Could you check a few things on this model? Use its own coordinates, in mm. Face numbers are marked on the shaded views. A direction names the side the tool comes from. Round coordinates to 2 decimals unless told otherwise and drop trailing zeros. Loops run counter-clockwise (first coordinate to the right, second up) from the corner with the lowest first, then second, coordinate; pieces in that order, holes last. Notation, with made-up numbers: M 60.25,70 L 85.25,70 A10 cw 85.25,75 Z; hole C 37.5,6.5 d8. An arc over 180 degrees is marked long. One line per item, written item: value. Start each with the question number.
Q1. Imagine slicing it at B-B (x = 8.75). Please give me the cut outline in (y, z).
Q2. Which directions (+Z, -Z, +X, -X, +Y, -Y) give clear straight access to the entire face, cutting with the end or side of a thin tool? Please do the marked faces 1, 2, 3, 4 and 5.
Q3. Imagine slicing it at A-A (z = 4.75). Please give me the cut outline in (x, y), then the cut area to 3 significant figures.
Q4. Please list where these lines run through material, in increasing order: line 1 along X through (y, z) = (7.5, 2.75); line 2 along X through (y, z) = (1.5, -0.5); line 3 along Y through (x, z) = (6.75, 1.5).
Q5. I'm going to push flat-ended pins straight in: pin 1 Ø3 at (x, y) = (7, 1.5) entering from -Z; pin 2 Ø1.5 at (y, z) = (3, 2.5) entering from -X; pin 3 Ø4 at (x, z) = (-7.5, -1.5) entering from +Y. Where does each tip first touch, or does it pass through?
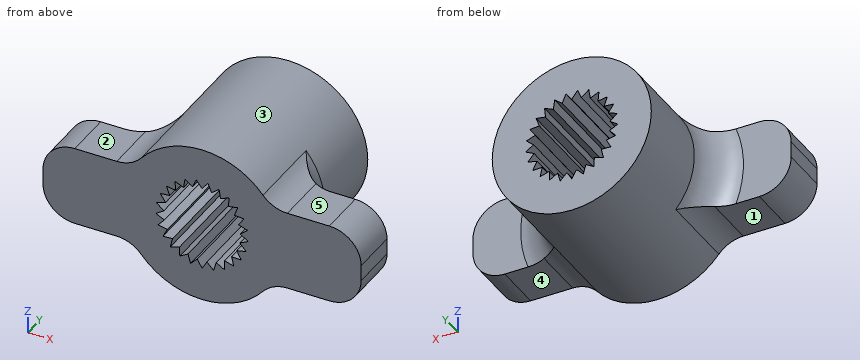
from build123d import *

# Parameters (mm, degrees)
SKETCH3_R           = 5
BOSS_EXTRUDE1_DEPTH = 10
SKETCH4_W           = 20
SKETCH4_H           = 5
BOSS_EXTRUDE2_DEPTH = 3
CUT_EXTRUDE1_DEPTH  = 11
FILLET2_R           = 2


with BuildPart() as part:
    # Sketch3 → Boss-Extrude1 (new body)
    with BuildSketch(Plane(origin=(0, 0, 0), x_dir=(1, 0, 0), z_dir=(0, 1, 0))):
        Circle(SKETCH3_R)
    extrude(amount=BOSS_EXTRUDE1_DEPTH)

    # Sketch4 → Boss-Extrude2 (add)
    with BuildSketch(Plane.XZ):
        Rectangle(SKETCH4_W, SKETCH4_H)
    extrude(amount=-BOSS_EXTRUDE2_DEPTH)

    # Sketch2 → Cut-Extrude1 (cut, through all)
    with BuildSketch(Plane(origin=(0, 0, 0), x_dir=(1, 0, 0), z_dir=(0, 1, 0))):
        Polygon((-0.302053093, 2.39099643), (0, 2.91), (0.302053093, 2.39099643), (0.723687572, 2.818576999), (0.887180172, 2.240761331), (1.401903192, 2.550052439), (1.416562458, 1.949730956), (1.992032078, 2.121298706), (1.856936915, 1.536191815), (2.456994263, 1.559255973), (2.180633196, 1.026128093), (2.767574462, 0.899239454), (2.367312274, 0.451588968), (2.90425778, 0.182720412), (2.405244416, -0.151325152), (2.8584559, -0.545279625), (2.292046204, -0.744730956), (2.633046723, -1.239017738), (2.0348303, -1.291342576), (2.242193536, -1.85490381), (1.649758525, -1.756814392), (1.710455084, -2.354239454), (1.161026355, -2.111899099), (1.071242448, -2.705649574), (0.599342628, -2.334285418), (0.36471971, -2.887053781), (0, -2.41), (-0.36471971, -2.887053781), (-0.599342628, -2.334285418), (-1.071242448, -2.705649574), (-1.161026355, -2.111899099), (-1.710455084, -2.354239454), (-1.649758525, -1.756814392), (-2.242193536, -1.85490381), (-2.0348303, -1.291342576), (-2.633046723, -1.239017738), (-2.292046204, -0.744730956), (-2.8584559, -0.545279625), (-2.405244416, -0.151325152), (-2.90425778, 0.182720412), (-2.367312274, 0.451588968), (-2.767574462, 0.899239454), (-2.180633196, 1.026128093), (-2.456994263, 1.559255973), (-1.856936915, 1.536191815), (-1.992032078, 2.121298706), (-1.416562458, 1.949730956), (-1.401903192, 2.550052439), (-0.887180172, 2.240761331), (-0.723687572, 2.818576999), align=None)
    extrude(amount=CUT_EXTRUDE1_DEPTH, mode=Mode.SUBTRACT)

    # Fillet2
    fillet2_edges = [part.edges().sort_by_distance(p)[0] for p in [
        (10, 1.5, -2.5),
        (-10, 1.5, 2.5),
        (10, 1.5, 2.5),
        (4.330127019, 1.5, -2.5),
        (-4.330127019, 1.5, -2.5),
        (-10, 1.5, -2.5),
        (-4.330127019, 1.5, 2.5),
        (4.330127019, 1.5, 2.5),
        (-5, 3, 0),
        (4.829629131, 3, -1.294095226),
    ]]
    fillet(fillet2_edges, radius=FILLET2_R)


solid = part.part
Report:
1. outline: M 0,-2.35 L 3,-2.35 L 3,2.35 L 0,2.35 Z
2. face 1: -Z, -X, +Y, -Y
2. face 2: +Z, -X, +Y, -Y
2. face 3: +Y
2. face 4: -Z, +X, +Y, -Y
2. face 5: +Z, +X, +Y, -Y
3. outline: M -1.56,0 L 1.56,0 L 1.56,10 L -1.56,10 Z
3. area: 31.2 mm²
4. line 1: x = -4.18 to -0.42, -0.26 to 0.26, 0.42 to 4.18
4. line 2: x = -10 to -2.41, 2.41 to 10
4. line 3: y = 0 to 3
5. pin 1: stops at z = -2.5
5. pin 2: stops at x = -9.56
5. pin 3: stops at y = 3.53
